Verification items for the finished model (mm, model axes). A direction names the side the tool comes from. Coordinates: 2 decimals unless noted, no trailing zeros. Loops run counter-clockwise (first coordinate to the right, second up) from the corner with the lowest first, then second, coordinate; pieces in that order, holes last. Notation, with made-up numbers: (75.25, -30.75) - (94.25, -30.75) arc R34 ccw to (94.25, 2.25) - close; hole circle Ø4 at (48, -36.5). An arc over 180 degrees is marked (long way). One line per item, written item: value. Start each with the question number.
(1) Section check D-D (y = 15.75). Record the boundary of the cut face in (x, z), plus the area to 3 significant figures.
(2) Section check B-B (x = 21.5). Record the boundary of the cut face in (y, z), plus the area to 3 significant figures.
(3) Gauge pin test, flat ends, axial feed: P1, Ø5.5, axis at x = 24.5, z = 7, coming from the -Y side; P2, Ø2, axis at x = 21, z = 8, coming from the +Y side; P3, Ø3, axis at x = 27.5, y = 3.5, coming from the +Z side. Record the tip position at first contact, or that the pin passes through.
(4) Draft check along Y on faces 1 (the face through (25, 8, 5)), 2 (the face through (25, 10, 7)), 3 (the face through (38.98, 2.39, 2.26)). Enter one of: +Y half, -Y half, draft (parallel to the pull), parting line (faces both ways), or undercut.
(5) Set-up check for faces 4 (the face through (8.59, 7.61, 6.55)), 5 (the face through (39.4, 1.7, 7)), 6 (the face through (12.5, 4.6, 9.2)): record each of +Z, -Z, +X, -X, +Y, -Y from which the full face is reachable in a straight line by a thin tool's end or side.
(6) Section check A-A (z = 2). Record the boundary of the cut face in (x, y).
(7) Thickness scan on probe 1 along X at (y, z) = (8.65, 7) (3 decimals); probe 2 along X at (y, z) = (16.25, 9.25); probe 3 along X at (y, z) = (3, 3.6). Record the ranges inside material, lowest first. Write a range as [from, to].
(8) Section check C-C (y = 5.5). Record the boundary of the cut face in (x, z), plus the area to 3 significant figures.
```python
from build123d import *

# Parameters (mm, degrees)
SKETCH_W             = 50
SKETCH_H             = 20
PAD_DEPTH            = 10
SKETCH001_W          = 42.5
SKETCH001_H          = 10
POCKET_DEPTH         = 7
SKETCH002_R          = 1.6
POCKET001_DEPTH      = 5
POCKET002_DEPTH      = 6.9
SKETCH004_R          = 1.6
POCKET003_DEPTH      = 10
SKETCH005_W          = 5.7
SKETCH005_H          = 2.6
POCKET004_DEPTH      = 6.15
SKETCH006_R          = 1.6
POCKET005_DEPTH      = 10
SKETCH007_R          = 8
PAD001_DEPTH         = 0.2
SKETCH008_R          = 4
POCKET006_DEPTH      = 2
POCKET006_DEPTH_BACK = -4
POCKET007_DEPTH      = 7


with BuildPart() as part:
    # Sketch → Pad (new body)
    with BuildSketch(Plane.XY):
        with Locations((25, 10)):
            Rectangle(SKETCH_W, SKETCH_H)
    extrude(amount=PAD_DEPTH)

    # Sketch001 (on Face6 of Pad) → Pocket (cut)
    with BuildSketch(Plane.XY.offset(10)):
        with Locations((25, 15)):
            Rectangle(SKETCH001_W, SKETCH001_H)
    extrude(amount=-POCKET_DEPTH, mode=Mode.SUBTRACT)

    # Sketch002 (on Face6 of Pocket) → Pocket001 (cut)
    with BuildSketch(Plane.XY.offset(3)):
        with Locations((10, 10)):
            Circle(SKETCH002_R)
        with Locations((40, 10)):
            Circle(SKETCH002_R)
    extrude(amount=-POCKET001_DEPTH, mode=Mode.SUBTRACT)

    # Sketch003 (on Face4 of Pocket001) → Pocket002 (cut)
    with BuildSketch(Plane.XY.offset(10)):
        Polygon((5.1, 0), (7.6, 6.1), (0, 6.1), (0, 0), align=None)
        Polygon((19.9, 0), (17.4, 6.1), (32.6, 6.1), (30.1, 0), align=None)
        Polygon((42.4, 6.1), (44.9, 0), (50, 0), (50, 6.1), align=None)
    extrude(amount=-POCKET002_DEPTH, mode=Mode.SUBTRACT)

    # Sketch004 (on Face4 of Pocket002) → Pocket003 (cut)
    with BuildSketch(Plane.XY.offset(10)):
        with Locations((12.5, 3)):
            Circle(SKETCH004_R)
        with Locations((37.5, 3)):
            Circle(SKETCH004_R)
    extrude(amount=-POCKET003_DEPTH, mode=Mode.SUBTRACT)

    # Sketch005 (on Face4 of Pocket003) → Pocket004 (cut)
    with BuildSketch(Plane.XY.offset(10)):
        with Locations((12.5, 3)):
            Rectangle(SKETCH005_W, SKETCH005_H)
        with Locations((37.5, 3)):
            Rectangle(SKETCH005_W, SKETCH005_H)
    extrude(amount=-POCKET004_DEPTH, mode=Mode.SUBTRACT)

    # Sketch006 (on Face9 of Pocket004) → Pocket005 (cut)
    with BuildSketch(Plane.XZ):
        with Locations((12.5, 7)):
            Circle(SKETCH006_R)
        with Locations((37.5, 7)):
            Circle(SKETCH006_R)
    extrude(amount=-POCKET005_DEPTH, mode=Mode.SUBTRACT)

    # Sketch007 (on Face2 of Pocket005) → Pad001 (join)
    with BuildSketch(Plane(origin=(0, 0, 0), x_dir=(1, 0, 0), z_dir=(0, 0, -1))):
        with Locations((25, -10)):
            Circle(SKETCH007_R)
    extrude(amount=PAD001_DEPTH)

    # Sketch008 (on Face47 of Pad001) → Pocket006 (cut, two sides)
    with BuildSketch(Plane(origin=(0, 0, 3), x_dir=(1, 0, 0), z_dir=(0, 0, -1))) as pocket006_sk:
        with Locations((25, -10)):
            Circle(SKETCH008_R)
    extrude(amount=-POCKET006_DEPTH, mode=Mode.SUBTRACT)
    extrude(pocket006_sk.sketch, amount=-POCKET006_DEPTH_BACK, mode=Mode.SUBTRACT)

    # Sketch009 (on Face4 of Pocket006) → Pocket007 (cut)
    with BuildSketch(Plane.XY.offset(10)):
        Polygon((12.775, 8.397853), (12.775, 11.602147), (10, 13.204294), (7.225, 11.602147), (7.225, 8.397853), (10, 6.795706), align=None)
        Polygon((42.775, 8.397853), (42.775, 11.602147), (40, 13.204294), (37.225, 11.602147), (37.225, 8.397853), (40, 6.795706), align=None)
    extrude(amount=-POCKET007_DEPTH, mode=Mode.SUBTRACT)


solid = part.part
```
Responses:
1. outline: (0, 0) - (19.44, 0) - (19.44, -0.2) - (30.56, -0.2) - (30.56, 0) - (50, 0) - (50, 10) - (46.25, 10) - (46.25, 3) - (3.75, 3) - (3.75, 10) - (0, 10) - close
1. area: 205 mm²
2. outline: (0, 0) - (2.81, 0) - (2.81, -0.2) - (8.06, -0.2) - (8.06, 5) - (10, 5) - (10, 10) - (6.1, 10) - (6.1, 3.1) - (0, 3.1) - close; (11.94, -0.2) - (17.19, -0.2) - (17.19, 0) - (20, 0) - (20, 3) - (11.94, 3) - close
2. area: 74.5 mm²
3. P1: stops at y = 6.1
3. P2: stops at y = 10
3. P3: stops at z = 3.1
4. face 1: draft
4. face 2: +Y half
4. face 3: undercut
5. face 4: +Z, +Y
5. face 5: +Z
5. face 6: +Z, -Z
6. outline: (0, 0) - (50, 0) - (50, 20) - (0, 20) - close; hole circle Ø3.2 at (10, 10); hole circle Ø3.2 at (12.5, 3); hole circle Ø8 at (25, 10); hole circle Ø3.2 at (37.5, 3); hole circle Ø3.2 at (40, 10)
7. probe 1: x = [0, 7.225], [14.1, 35.9], [42.775, 50]
7. probe 2: x = [0, 3.75], [46.25, 50]
7. probe 3: x = [6.33, 10.9], [14.1, 18.67], [31.33, 35.9], [39.1, 43.67]
8. outline: (0, 0) - (18.39, 0) - (18.39, -0.2) - (31.61, -0.2) - (31.61, 0) - (50, 0) - (50, 3.1) - (42.65, 3.1) - (42.65, 10) - (32.35, 10) - (32.35, 3.1) - (17.65, 3.1) - (17.65, 10) - (7.35, 10) - (7.35, 3.1) - (0, 3.1) - close; hole circle Ø3.2 at (12.5, 7); hole circle Ø3.2 at (37.5, 7)
8. area: 284 mm²
